Part model, mm, in its own coordinate system. A direction names the side the tool comes from. Round coordinates to 2 decimals unless told otherwise and drop trailing zeros. Write each loop counter-clockwise with the first axis right and the second up, starting at its lowest first coordinate (ties: lowest second). Pieces come first, ordered by that corner, then holes.
from build123d import *

# Parameters (mm, degrees)
SKETCH1_W           = 50
SKETCH1_H           = 85
SKETCH1_R           = 1.375
BOSS_EXTRUDE1_DEPTH = 1.6
FILLET1_R           = 3.5
SKETCH5_W           = 5
SKETCH5_H           = 51
BOSS_EXTRUDE3_DEPTH = 10
BOSS_EXTRUDE4_DEPTH = 3


with BuildPart() as part:
    # Sketch1 → Boss-Extrude1 (new body)
    with BuildSketch(Plane(origin=(0, 0, 0), x_dir=(1, 0, 0), z_dir=(0, 1, 0))):
        with Locations((25, 42.5)):
            Rectangle(SKETCH1_W, SKETCH1_H)
        with Locations(Location((3.5, 3.5, 0), (0, 0, 270))):
            Circle(SKETCH1_R, mode=Mode.SUBTRACT)
        with Locations(Location((47.5, 3.5, 0), (0, 0, 270))):
            Circle(SKETCH1_R, mode=Mode.SUBTRACT)
        with Locations(Location((47.5, 61.5, 0), (0, 0, 270))):
            Circle(SKETCH1_R, mode=Mode.SUBTRACT)
        with Locations(Location((3.5, 61.5, 0), (0, 0, 270))):
            Circle(SKETCH1_R, mode=Mode.SUBTRACT)
    extrude(amount=BOSS_EXTRUDE1_DEPTH)

    # Fillet1
    fillet1_edges = [part.edges().sort_by_distance(p)[0] for p in [
        (0, 0.8, -85),
        (50, 0.8, -85),
        (50, 0.8, 0),
        (0, 0.8, 0),
    ]]
    fillet(fillet1_edges, radius=FILLET1_R)

    # Sketch5 → Boss-Extrude3 (add)
    with BuildSketch(Plane(origin=(0, 1.6, 0), x_dir=(1, 0, 0), z_dir=(0, 1, 0))):
        with Locations((3.5, 32.5)):
            Rectangle(SKETCH5_W, SKETCH5_H)
    extrude(amount=BOSS_EXTRUDE3_DEPTH)

    # Sketch6 → Boss-Extrude4 (add)
    with BuildSketch(Plane(origin=(0, 1.6, 0), x_dir=(1, 0, 0), z_dir=(0, 1, 0))):
        Polygon((26.64840561, 57.006203003), (38.214146185, 45.322359626), (26.383805878, 33.611602944), (14.818065303, 45.295446321), align=None)
    extrude(amount=BOSS_EXTRUDE4_DEPTH)


solid = part.part
Q1. Saw through at A-A, the plane z = -61.5. Write the cut outline in (x, y) (3 decimals).
Q2. Wall check: line 1 (Y direction, x = 16, z = -17); line 2 (Z direction, x = 5, y = 8.25); line 3 (X direction, y = 7.5, z = -12.5). Give the ranges that are in metal, low to high.
Q3. Drop flat-ended pins along their axis: P1, Ø5, axis at y = 5, z = -21.5, coming from the -X side; P2, Ø1.5, axis at x = 3.5, y = 4.5, coming from the +Z side; P3, Ø7, axis at x = 21.5, z = -44, coming from the +Y side; P4, Ø1.5, axis at x = 28, y = 6, coming from the -Z side. Give the stop position or say it passes through.
Q4. Two-plate mould, pull along Z, no slides. Class faces 4 (the flat face through (32.38, 3.08, -39.55)), 5 (the cylindrical face through (46.16, 0.79, -3.8)), 6 (the flat face through (6, 7, -32)): released by +Z, released by -Z, zero draft, split by the parting line, or undercut.
Q5. Tool access for faces 1 (the flat face through (20.65, 3.08, -51.07)), 2 (the flat face through (3, 7, -7)), 3 (the flat face through (32.35, 3.079, -51.246)): list every direction of +Z, -Z, +X, -X, +Y, -Y with a clear straight run to the whole face (end or side of a thin tool).
Q6. Saw through at C-C, the plane y = 7. Write the cut outline in (x, z), and give its area (3 significant figures).
Q7. Saw through at D-D, the plane z = -22. Write the cut outline in (x, y).
Q8. Saw through at B-B, the plane x = 47.5. Write the cut outline in (y, z) (3 decimals).
Computed:
1. outline: (0, 0) - (2.125, 0) - (2.125, 1.6) - (0, 1.6) - close; (4.875, 0) - (46.125, 0) - (46.125, 1.6) - (4.875, 1.6) - close; (48.875, 0) - (50, 0) - (50, 1.6) - (48.875, 1.6) - close
2. line 1: y = 0 to 1.6
2. line 2: z = -58 to -7
2. line 3: x = 1 to 6
3. P1: stops at x = 1
3. P2: stops at z = -7
3. P3: stops at y = 4.6
3. P4: passes through
4. face 4: released by +Z
4. face 5: undercut
4. face 6: zero draft
5. face 1: -Z, +Y
5. face 2: +Z, +X, -X, +Y
5. face 3: -Z, +X, +Y
6. outline: (1, -58) - (6, -58) - (6, -7) - (1, -7) - close
6. area: 255 mm2
7. outline: (0, 0) - (50, 0) - (50, 1.6) - (6, 1.6) - (6, 11.6) - (1, 11.6) - (1, 1.6) - (0, 1.6) - close
8. outline: (0, -84.854) - (1.6, -84.854) - (1.6, -62.875) - (0, -62.875) - close; (0, -60.125) - (1.6, -60.125) - (1.6, -4.875) - (0, -4.875) - close; (0, -2.125) - (1.6, -2.125) - (1.6, -0.146) - (0, -0.146) - close
